from build123d import *

# Parameters (mm, degrees)
SKETCH1_W               = 152.4
SKETCH1_H               = 304.8
BOSS_EXTRUDE1_DEPTH     = 6.35
F_1_4_20_TAPPED_HOLE1_D = 5.1054
LPATTERN1_COUNT         = 4
LPATTERN1_PITCH         = 76.2


with BuildPart() as part:
    # Sketch1 → Boss-Extrude1 (new body)
    with BuildSketch(Plane(origin=(0, 0, 0), x_dir=(1, 0, 0), z_dir=(0, 1, 0))):
        with Locations((76.2, 0)):
            Rectangle(SKETCH1_W, SKETCH1_H)
    extrude(amount=BOSS_EXTRUDE1_DEPTH)

    # 1/4-20 Tapped Hole1 (through all)
    with Locations(Plane(origin=(0, 6.35, 0), x_dir=(1, 0, 0), z_dir=(0, 1, 0))):
        with Locations((130.5, 137.4), (108, 115.175), (108, -2.6), (108, -56.575), (108, 89.775)):
            Hole(F_1_4_20_TAPPED_HOLE1_D / 2)

    # Sketch4 → 1/4 Clearance Hole2 (revolve, cut)
    with BuildSketch(Plane(origin=(139.7, 6.35, -114.3), x_dir=(0, 0, 1), z_dir=(1, 0, 0))):
        Polygon((0, 0), (0, 14.845817477), (3.57124, 12.7), (3.57124, 0), align=None)
    f_1_4_clearance_hole2 = revolve(axis=Axis((139.7, 12.7, -114.3), (0, -1, 0)), mode=Mode.SUBTRACT)

    # LPattern1: 1/4 Clearance Hole2 ×4
    with Locations(*[(0, 0, i * LPATTERN1_PITCH) for i in range(1, LPATTERN1_COUNT)]):
        add(f_1_4_clearance_hole2, mode=Mode.SUBTRACT)

    # Mirror1: part across plane


with BuildPart() as part_1:
    add(part.part)
    add(part.part.mirror(Plane(origin=(0, 0, 0), x_dir=(0, 0, 1), z_dir=(1, 0, 0))))


solid = part_1.part
For this review, take the finished solid that the model builds, in its own axes (mm). Coordinates: 2 decimals unless noted, no trailing zeros. Loops run counter-clockwise (first coordinate to the right, second up) from the corner with the lowest first, then second, coordinate; pieces in that order, holes last. Notation, with made-up numbers: (-27.5, 14) - (20.5, 14) arc R13 ccw to (20.5, 23) - close; hole circle Ø8 at (54.5, 45). An arc over 180 degrees is marked (long way). Use a Markdown table: item, result. Add a question column.
Item 1: For line 1 (Z direction, x = 139.7, y = 2.5); line 2 (X direction, y = 2, z = 114.3); line 3 (Z direction, x = -130.5, y = 1.5), list the stretches that pass through material, from the lowest coordinate up.
Item 2: We need section A-A (x = -139.7). Give the boundary of the cut face in (y, z), and give its area (3 significant figures).
Item 3: Insertion check: pin 1 Ø5.5 at (x, z) = (139.7, -114.3) entering from +Y. The pin has a flat end and moves straight along its axis. Give the tip position at first contact, or say it passes through.
Item 4: We need section B-B (z = 38.1). Give the boundary of the cut face in (x, y).
Item 5: Mouldability with a two-part tool opening along X and no side actions: class faces 1 (the face through (136.16, 3.22, 37.64)), 2 (the face through (2, 0, -2)) as pulls with the +X half, pulls with the -X half, needs draft (parallel to the pull), parting line crosses it, or undercut.
Results list:
| question | item | result |
|---|---|---|
| 1 | line 1 | z = -152.4 to -117.87, -110.73 to -41.67, -34.53 to 34.53, 41.67 to 110.73, 117.87 to 152.4 |
| 1 | line 2 | x = -152.4 to -143.27, -136.13 to 136.13, 143.27 to 152.4 |
| 1 | line 3 | z = -152.4 to -139.95, -134.85 to 152.4 |
| 2 | outline | (0, -152.4) - (6.35, -152.4) - (6.35, -117.87) - (0, -117.87) - close; (0, -110.73) - (6.35, -110.73) - (6.35, -41.67) - (0, -41.67) - close; (0, -34.53) - (6.35, -34.53) - (6.35, 34.53) - (0, 34.53) - close; (0, 41.67) - (6.35, 41.67) - (6.35, 110.73) - (0, 110.73) - close; (0, 117.87) - (6.35, 117.87) - (6.35, 152.4) - (0, 152.4) - close |
| 2 | area | 1,750 mm^2 |
| 3 | pin 1 | passes through |
| 4 | outline | (-152.4, 0) - (-143.27, 0) - (-143.27, 6.35) - (-152.4, 6.35) - close; (-136.13, 0) - (136.13, 0) - (136.13, 6.35) - (-136.13, 6.35) - close; (143.27, 0) - (152.4, 0) - (152.4, 6.35) - (143.27, 6.35) - close |
| 5 | face 1 | undercut |
| 5 | face 2 | needs draft |
